Can you work these out from the drawing? Everything is in mm from the part's minimum corner. A direction names the side the tool comes from. Coordinates: 2 decimals unless noted, no trailing zeros. Order: outer loops, then holes, each group sorted by start corner. A loop starts at its lowest first (then second) coordinate and runs counter-clockwise, first axis right, second up. Notation, with made-up numbers: M 22,9 L 49,9 A14 ccw 49,19 Z; hole C 2,16.25 d3. An arc over 180 degrees is marked long. Answer as CSV lines item,"result". Start each with the question number.
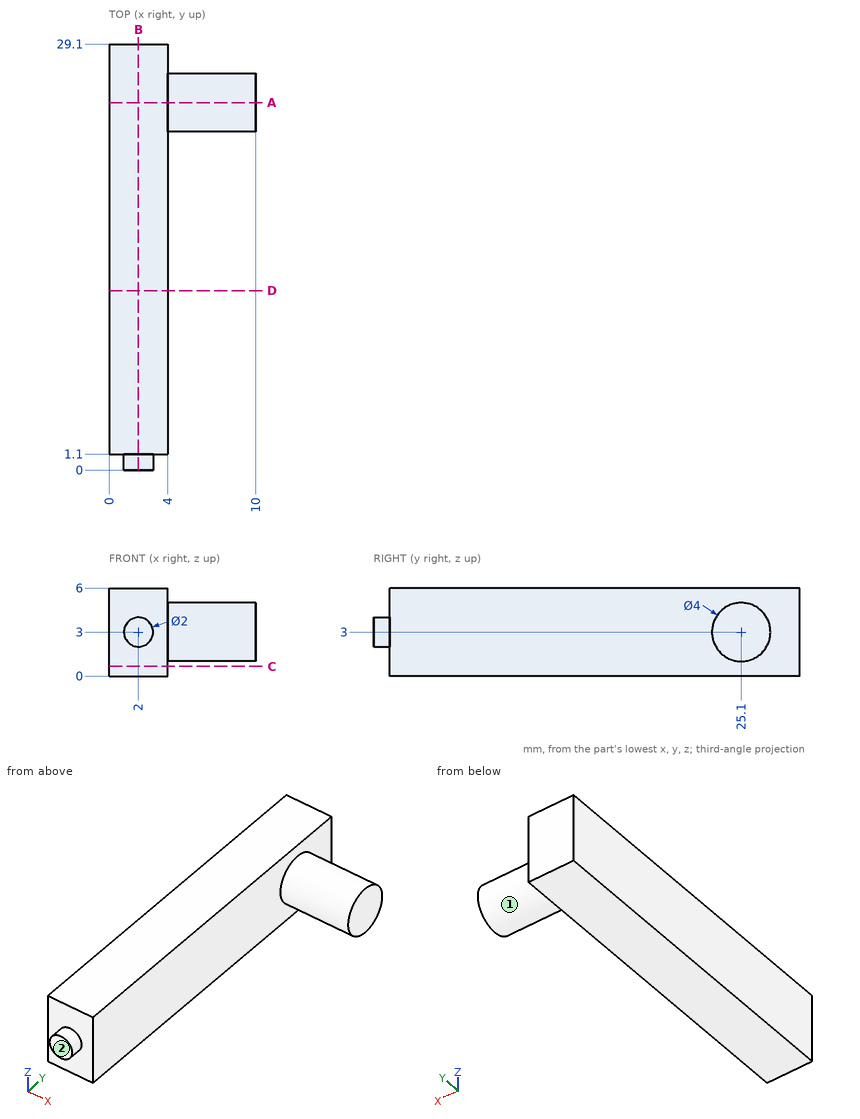
1) I need wall thicknesses on line 1 (Y direction, x = 1.5, z = 3.9); line 2 (X direction, y = 19.75, z = 5.2); line 3 (Z direction, x = 8.5, y = 24.5). Which ranges of each line are inside material? Lowest first, please. Write a range as [from, to].
2) Suppose I cut it at B-B on x = 2. Please give me the cut outline in (y, z).
3) Suppose I cut it at C-C on z = 0.65. Please give me the cut outline in (x, y).
4) Will these pins go through, and if not, where does the flat tip stop? pin 1 Ø2 at (x, z) = (6.5, 5) entering from +Y; pin 2 Ø1.5 at (y, z) = (6.5, 1) entering from +X.
5) Suppose I cut it at A-A on y = 25.1. Please give me the cut outline in (x, z), plus the area to 3 significant figures.
6) Which directions (+Z, -Z, +X, -X, +Y, -Y) give clear straight access to the entire face, cutting with the end or side of a thin tool? Please do the marked faces 1 and 2.
7) Suppose I cut it at D-D on y = 12.25. Please give me the cut outline in (x, z).
Output:
1,line 1,"[1.1, 29.1]"
1,line 2,"[0, 4]"
1,line 3,"[1.09, 4.91]"
2,outline,"M 0,2 L 1.1,2 L 1.1,0 L 29.1,0 L 29.1,6 L 1.1,6 L 1.1,4 L 0,4 Z"
3,outline,"M 0,1.1 L 4,1.1 L 4,29.1 L 0,29.1 Z"
4,pin 1,"y = 26.83"
4,pin 2,"x = 4"
5,outline,"M 0,0 L 4,0 L 4,1 L 10,1 L 10,5 L 4,5 L 4,6 L 0,6 Z"
5,area,"48.0 mm²"
6,face 1,"+X"
6,face 2,"+Z, -Z, +X, -X, -Y"
7,outline,"M 0,0 L 4,0 L 4,6 L 0,6 Z"
